Input: part model. Units: mm. Frame: model coordinates. Face numbers are marked on the shaded views. A direction names the side the tool comes from. Round coordinates to 2 decimals unless told otherwise and drop trailing zeros. Loops run counter-clockwise (first coordinate to the right, second up) from the corner with the lowest first, then second, coordinate; pieces in that order, holes last. Notation, with made-up numbers: (19.5, 42) - (25.5, 42) arc R10 cw to (25.5, 52) - close; hole circle Ø9 at (-3.75, 80). An arc over 180 degrees is marked (long way). Use CSV: the item, a comma, the result in double quotes. Start each with the question number.
1. Material intervals for probe 1 along Y at (x, z) = (-0.15, -2.7); probe 2 along X at (y, z) = (3.05, -2); probe 3 along Z at (x, y) = (-0.1, -0.25), sorted ascending. Write a range as from..to.
2. Pull-direction query (Y, two-part tool) for the marked faces 1, 2 and 3; classes: +Y half, -Y half, draft (parallel to the pull), parting line (faces both ways), or undercut.
3. Access query for the marked faces 4, 5, 6, 7 and 8. Directions: +Z, -Z, +X, -X, +Y, -Y. A direction counts if a zero-diameter tool reaches every point of the face in a straight line with its end or side. Return the directions, or none.
4. Pin query (flat end, axial travel): P1, Ø1, axis at x = 0.5, y = -1, coming from the -Z side; P2, Ø0.7, axis at x = 0, y = 0, coming from the +Z side. Return the tip coordinate at first contact, or that it passes through.
5. Cut plane A-A (z = -0.55). Return loops of the section in (x, y).
6. Cut plane C-C (z = -1.9). Return loops of the section in (x, y), and give its area (3 significant figures).
7. Cut plane B-B (x = 0). Return loops of the section in (y, z) (3 decimals), and give its area (3 significant figures).
8. Cut plane D-D (y = -0.5). Return loops of the section in (x, z), and give its area (3 significant figures).
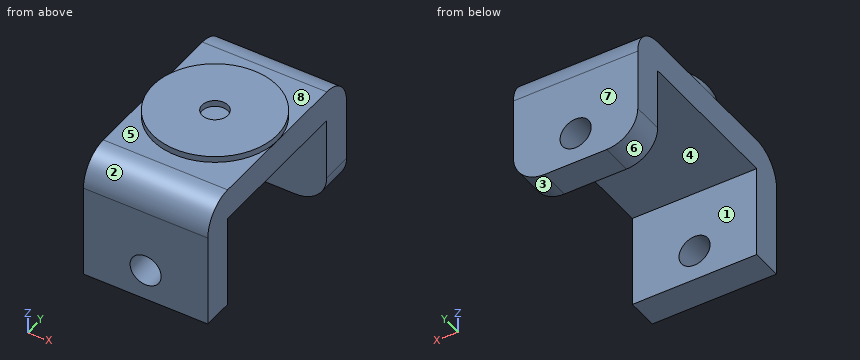
```python
from build123d import *

# Parameters (mm, degrees)
SKETCH1_W           = 4
SKETCH1_H           = 5
BOSS_EXTRUDE1_DEPTH = 1
SKETCH2_W           = 4
SKETCH2_H           = 1
BOSS_EXTRUDE2_DEPTH = 2
FILLET1_R           = 1
SKETCH3_R           = 2
SKETCH3_R_2         = 0.415
BOSS_EXTRUDE3_DEPTH = 0.2
SKETCH4_R           = 0.5
CUT_EXTRUDE1_DEPTH  = 8.874007874


with BuildPart() as part:
    # Sketch1 → Boss-Extrude1 (new body)
    with BuildSketch(Plane.XY):
        Rectangle(SKETCH1_W, SKETCH1_H)
    extrude(amount=BOSS_EXTRUDE1_DEPTH)

    # Sketch2 → Boss-Extrude2 (add, symmetric)
    with BuildSketch(Plane(origin=(0, 0, 0), x_dir=(0, 0, -1), z_dir=(1, 0, 0))):
        with Locations((1, 3)):
            Rectangle(SKETCH2_W, SKETCH2_H)
        with Locations((1, -3)):
            Rectangle(SKETCH2_W, SKETCH2_H)
    extrude(amount=BOSS_EXTRUDE2_DEPTH, both=True)

    # Fillet1
    fillet1_edges = [part.edges().sort_by_distance(p)[0] for p in [
        (0, 3.5, 1),
        (-2, 3, -3),
        (2, 3, -3),
        (0, -3.5, 1),
    ]]
    fillet(fillet1_edges, radius=FILLET1_R)

    # Sketch3 → Boss-Extrude3 (add)
    with BuildSketch(Plane.XY.offset(1)):
        Circle(SKETCH3_R)
        Circle(SKETCH3_R_2, mode=Mode.SUBTRACT)
    extrude(amount=BOSS_EXTRUDE3_DEPTH)

    # Sketch4 → Cut-Extrude1 (cut, through all)
    with BuildSketch(Plane.XZ.offset(3.5)):
        with Locations(Location((0, -2, 0), (0, 0, 270))):
            Circle(SKETCH4_R)
    extrude(amount=-CUT_EXTRUDE1_DEPTH, mode=Mode.SUBTRACT)


solid = part.part
```
Established:
1,probe 1,"y = -3.5..-2.5, 2.5..3.5"
1,probe 2,"x = -2..-0.5, 0.5..2"
1,probe 3,"z = 0..1"
2,face 1,"undercut"
2,face 2,"-Y half"
2,face 3,"draft"
3,face 4,"-Z, +X, -X"
3,face 5,"+Z, -Y"
3,face 6,"-Z, -X, +Y"
3,face 7,"+Z, -Z, +X, -X, +Y"
3,face 8,"+Z, +Y"
4,P1,"stops at z = 0"
4,P2,"stops at z = 1"
5,outline,"(-2, -3.5) - (2, -3.5) - (2, -2.5) - (-2, -2.5) - close; (-2, 2.5) - (2, 2.5) - (2, 3.5) - (-2, 3.5) - close"
6,outline,"(-2, -3.5) - (-0.49, -3.5) - (-0.49, -2.5) - (-2, -2.5) - close; (-2, 2.5) - (-0.49, 2.5) - (-0.49, 3.5) - (-2, 3.5) - close; (0.49, -3.5) - (2, -3.5) - (2, -2.5) - (0.49, -2.5) - close; (0.49, 2.5) - (2, 2.5) - (2, 3.5) - (0.49, 3.5) - close"
6,area,"6.04 mm2"
7,outline,"(-3.5, -3) - (-2.5, -3) - (-2.5, -2.5) - (-3.5, -2.5) - close; (-3.5, -1.5) - (-2.5, -1.5) - (-2.5, 0) - (2.5, 0) - (2.5, -1.5) - (3.5, -1.5) - (3.5, 0) arc R1 ccw to (2.5, 1) - (2, 1) - (2, 1.2) - (0.415, 1.2) - (0.415, 1) - (-0.415, 1) - (-0.415, 1.2) - (-2, 1.2) - (-2, 1) - (-2.5, 1) arc R1 ccw to (-3.5, 0) - close; (2.5, -3) - (3.5, -3) - (3.5, -2.5) - (2.5, -2.5) - close"
7,area,"11.2 mm2"
8,outline,"(-2, 0) - (2, 0) - (2, 1) - (1.94, 1) - (1.94, 1.2) - (-1.94, 1.2) - (-1.94, 1) - (-2, 1) - close"
8,area,"4.77 mm2"
